from build123d import *

# Parameters (mm, degrees)
SKETCH_1_R      = 18.5
SKETCH_1_R_2    = 13
EXTRUDE_1_DEPTH = 15


with BuildPart() as part:
    # 草图1 → 凸台-拉伸1 (new body)
    with BuildSketch(Plane(origin=(0, 0, 0), x_dir=(1, 0, 0), z_dir=(0, 1, 0))):
        with BuildLine():
            Line((65.196415688, 20.938478113), (339.27978891, 27.990735896))
            ThreePointArc((339.27978891, 27.990735896), (368, 0), (339.27978891, -27.990735896))
            Line((339.27978891, -27.990735896), (65.196415688, -20.938478113))
            ThreePointArc((65.196415688, -20.938478113), (39.495702891, -23.306065445), (15.054107063, -31.597054618))
            ThreePointArc((15.054107063, -31.597054618), (-35, 0), (15.054107063, 31.597054618))
            ThreePointArc((15.054107063, 31.597054618), (39.495702891, 23.306065445), (65.196415688, 20.938478113))
        make_face()
        with Locations(Location((0, 0, 0), (0, 0, 270))):
            Circle(SKETCH_1_R, mode=Mode.SUBTRACT)
        with Locations(Location((340, 0, 0), (0, 0, 270))):
            Circle(SKETCH_1_R_2, mode=Mode.SUBTRACT)
    extrude(amount=EXTRUDE_1_DEPTH)


solid = part.part
Part model, mm, in its own coordinate system. A direction names the side the tool comes from. Give positions to 0.01 mm unless a question says otherwise; leave off trailing zeros. Loops run counter-clockwise (first coordinate to the right, second up) from the corner with the lowest first, then second, coordinate; pieces in that order, holes last. Notation, with made-up numbers: M -7,-35.5 L 6,-35.5 A21 ccw 6,-9.5 Z; hole C 17,49.5 d5. An arc over 180 degrees is marked long. Put each result on its own line as item: value. Start each with the question number.
1) Probe probe 1 along X at (y, z) = (8.5, 0); probe 2 along X at (y, z) = (3.75, -9); probe 3 along Z at (x, y) = (-10.5, 2.75). List the from-to ranges inside material, lowest first.
2) Saw through at B-B (z = 0). List the corners of the cut face in (x, y).
3) Saw through at A-A (x = 0). List the corners of the cut face in (y, z).
4) Pull direction X, two halves, no side cores. Call faces 1 (the flat face through (169, 0, 0)), 2 (the cylindrical face through (39.85, 7.4, 23.23)), 3 (the cylindrical face through (-34.986, 7.395, 0.987)): +X half, -X half, draft (parallel to the pull), parting line (faces both ways), or undercut.
5) Flat gauge pins, fed straight in: pin 1 (4 mm diameter, centred on x = 200, y = 11, fed in from -Z); pin 2 (6 mm diameter, centred on x = 311.5, y = 8.5, fed in from -Z); pin 3 (1 mm diameter, centred on y = 4, z = -4, fed in from +X); pin 4 (15.5 mm diameter, centred on x = 340, z = 0, fed in from -Y). Where does each tip first touch, or does it go through?
6) 3-axis set-ups, long thin cutter, end or side, ignore diameter. For faces 4 (the cylindrical face through (39.142, 7.395, -23.382)), 5 (the flat face through (169, 15, 0)): which of +Z, -Z, +X, -X, +Y, -Y reach the whole face in a straight line?
7) Saw through at C-C (y = 6). List the corners of the cut face in (x, z).
8) Saw through at D-D (x = 331). List the corners of the cut face in (y, z), then the cut area to 3 significant figures.
Numbers:
1. probe 1: -35 to -18.5, 18.5 to 327, 353 to 368
1. probe 2: -33.82 to -16.16, 16.16 to 330.62, 349.38 to 366.51
1. probe 3: -33.39 to -15.23, 15.23 to 33.39
2. outline: M -35,0 L -18.5,0 L -18.5,15 L -35,15 Z; M 18.5,0 L 327,0 L 327,15 L 18.5,15 Z; M 353,0 L 368,0 L 368,15 L 353,15 Z
3. outline: M 0,-35 L 15,-35 L 15,-18.5 L 0,-18.5 Z; M 0,18.5 L 15,18.5 L 15,35 L 0,35 Z
4. face 1: draft
4. face 2: undercut
4. face 3: parting line
5. pin 1: z = -24.46
5. pin 2: z = -27.35
5. pin 3: x = 367.78
5. pin 4: through
6. face 4: -Z, +Y, -Y
6. face 5: +Z, -Z, +X, -X, +Y
7. outline: M 15.05,-31.6 A110 cw 65.2,-20.94 L 339.28,-27.99 A28 ccw long 339.28,27.99 L 65.2,20.94 A110 cw 15.05,31.6 A35 ccw long Z; hole C 0,0 d37; hole C 340,0 d26
8. outline: M 0,-27.78 L 15,-27.78 L 15,-9.38 L 0,-9.38 Z; M 0,9.38 L 15,9.38 L 15,27.78 L 0,27.78 Z
8. area: 552 mm^2
